```python
from build123d import *

# Parameters (mm, degrees)
SKETCH1_W           = 22.225
SKETCH1_H           = 22.225
BOSS_EXTRUDE1_DEPTH = 254
SKETCH4_R           = 2.38125
CUT_EXTRUDE2_DEPTH  = 26.4
SKETCH6_R           = 2.4892
CUT_EXTRUDE3_DEPTH  = 25.4


with BuildPart() as part:
    # Sketch1 → Boss-Extrude1 (new body)
    with BuildSketch(Plane(origin=(0, 0, 0), x_dir=(-1, 0, 0), z_dir=(0, 0, -1))):
        with BuildLine():
            Line((1.5875, -1.3335), (1.5875, 23.5585))
            ThreePointArc((1.5875, 23.5585), (1.513105122, 23.738105122), (1.3335, 23.8125))
            Line((1.3335, 23.8125), (-23.5585, 23.8125))
            ThreePointArc((-23.5585, 23.8125), (-23.738105122, 23.738105122), (-23.8125, 23.5585))
            Line((-23.8125, 23.5585), (-23.8125, -1.3335))
            ThreePointArc((-23.8125, -1.3335), (-23.738105122, -1.513105122), (-23.5585, -1.5875))
            Line((-23.5585, -1.5875), (1.3335, -1.5875))
            ThreePointArc((1.3335, -1.5875), (1.513105122, -1.513105122), (1.5875, -1.3335))
        make_face()
        with Locations((-11.1125, 11.1125)):
            Rectangle(SKETCH1_W, SKETCH1_H, mode=Mode.SUBTRACT)
    extrude(amount=-BOSS_EXTRUDE1_DEPTH)

    # Sketch4 → Cut-Extrude2 (cut, through all)
    with BuildSketch(Plane(origin=(23.8125, 0, 0), x_dir=(0, 0, -1), z_dir=(1, 0, 0))):
        with Locations((-37.933268304, 11.1125)):
            Circle(SKETCH4_R)
    extrude(amount=-CUT_EXTRUDE2_DEPTH, mode=Mode.SUBTRACT)

    # Sketch6 → Cut-Extrude3 (cut)
    with BuildSketch(Plane(origin=(0, 23.8125, 0), x_dir=(1, 0, 0), z_dir=(0, 1, 0))):
        with Locations((11.1125, -203.2)):
            Circle(SKETCH6_R)
        with Locations((11.1125, -228.6)):
            Circle(SKETCH6_R)
    extrude(amount=-CUT_EXTRUDE3_DEPTH, mode=Mode.SUBTRACT)


solid = part.part
```
Could you check a few things on this model? Use its own coordinates, in mm. A direction names the side the tool comes from. Coordinates: 2 decimals unless noted, no trailing zeros. Loops run counter-clockwise (first coordinate to the right, second up) from the corner with the lowest first, then second, coordinate; pieces in that order, holes last.
1) Will this pin go through, and if not, where does the flat tip stop? pin 1 Ø1.5 at (x, y) = (20, 9) entering from +Z.
Reported:
pin 1: passes through
2) Imagine slicing it at A-A (y = 6.5). List the corners of the cut face in (x, z) for me (1 decimal), and give its area (3 significant figures).
Reported:
outline: (-1.6, 0) - (0, 0) - (0, 254) - (-1.6, 254) - close; (22.2, 0) - (23.8, 0) - (23.8, 254) - (22.2, 254) - close
area: 806 mm2
3) Please list where these lines run through material, in increasing order: line 1 along X through (y, z) = (17.75, 125) (1 decimal); line 2 along X through (y, z) = (23.35, 228.6).
Reported:
line 1: x = -1.6 to 0, 22.2 to 23.8
line 2: x = -1.59 to 8.62, 13.6 to 23.81
4) Which directions (+Z, -Z, +X, -X, +Y, -Y) give clear straight access to the entire face, cutting with the end or side of a thin tool? Please do faces 4 (the face through (11, 0, 125)), 5 (the face through (23.812, 11, 125)).
Reported:
face 4: +Z, -Z
face 5: +Z, -Z, +X, +Y, -Y
5) Thinking about a two-plate mould opening in Z: for faces 1 (the face through (11, -1.588, 125)), 2 (the face through (10.57, -0.78, 205.63)), 3 (the face through (22.5, 11.2, 0)), which applies, released by +Z, released by -Z, zero draft, split by the parting line, or undercut?
Reported:
face 1: zero draft
face 2: undercut
face 3: released by -Z
